Read the model definition and answer for the solid it produces. Units are mm, in the model's axes. Coordinates: 2 decimals unless noted, no trailing zeros. Write each loop counter-clockwise with the first axis right and the second up, starting at its lowest first coordinate (ties: lowest second). Pieces come first, ordered by that corner, then holes. Notation, with made-up numbers: (45.5, 1.5) -> (93.5, 1.5) arc R35 ccw to (93.5, 38.5) -> close; hole circle Ø8 at (17, 55.5). An arc over 180 degrees is marked (long way). Write item = value, one per line. Start each with the question number.
1) For a pull along Y with two mould halves and no side action, classify faces 1 (the face through (9, 0, 3.175)), 2 (the face through (13.45, 0.24, 1.61)), 3 (the face through (26.034, 0.092, 1.565)) as released by +Y, released by -Y, zero draft, split by the parting line, or undercut.
2) Section D-D (y = -2.25) is taken. Determine the outline of the cut face in (x, z) (3 decimals).
3) Section A-A (z = 2.6) is taken. Determine the outline of the cut face in (x, y).
4) Flat-ended cylindrical pins translate along their axes: pin 1 Ø1.4 at (x, y) = (18.796, 0) entering from +Z; pin 2 Ø3 at (x, y) = (19, 0.5) entering from -Z; pin 3 Ø1.5 at (x, z) = (7.5, 2.5) entering from +Y. Find the tip coordinate at first contact, or state that the pin passes through.
5) Find the intervals of material crossed by line 1 along Y through (x, z) = (12.7, 1); line 2 along X through (y, z) = (-1, 2.6); line 3 along Y through (x, z) = (-2, 1.05), in increasing order. Write a range as from..to.
6) Section C-C (x = 12.5) is taken. Determine the outline of the cut face in (y, z) (3 decimals), plus the area to 3 significant figures.
7) Section B-B (y = 0) is taken. Determine the outline of the cut face in (x, z) (3 decimals), plus the area to 3 significant figures.
Autodesk Inventor part; units mm, degrees
ref_plane "YZ Plane" through (0, 0, 0) normal (1, 0, 0) x (0, 1, 0)
ref_plane "XZ Plane" through (0, 0, 0) normal (0, 1, 0) x (-1, 0, 0)
ref_plane "XY Plane" through (0, 0, 0) normal (0, 0, 1) x (1, 0, 0)
sketch "Sketch1" plane through (0, 0, 0) normal (0, 0, 1) x (1, 0, 0)
  circle A0 centre (0, 0) radius 6.9469
  circle A1 centre (21.844, 0) radius 4.191
  line L0 (0, 6.9469) -> (21.844, 4.191)
  line L1 (0, -6.9469) -> (21.844, -4.191)
  dimension "d0" = 13.8938
  dimension "d1" = 8.382
  dimension "d2" = 21.844
extrude "Extrusion1" add sketch "Sketch1" along normal blind 3.175 contours L0 A0 L1 | L0 A1 L1 A0 | A1
sketch "Sketch2" plane through (0, 0, 3.175) normal (0, 0, 1) x (1, 0, 0)
  circle A0 centre (0, 0) radius 2.54
  circle A1 centre (12.7, 0) radius 0.7874
  circle A2 centre (15.748, 0) radius 0.7874
  circle A3 centre (18.796, 0) radius 0.7874
  circle A4 centre (21.844, 0) radius 0.7874
  dimension "d5" = 5.08
  dimension "d6" = 1.5748
  dimension "d7" = 1.5748
  dimension "d8" = 1.5748
  dimension "d9" = 1.5748
  dimension "d10" = 12.7
  dimension "d11" = 15.748
  dimension "d12" = 18.796
  dimension "d13" = 21.844
extrude "Extrusion2" cut sketch "Sketch2" against normal blind 3.175
properties part number "Servo horn"
Answer key:
q1.face_1 = zero draft
q1.face_2 = undercut
q1.face_3 = split by the parting line
q2.outline = (-6.572, 0) -> (-1.179, 0) -> (-1.179, 3.175) -> (-6.572, 3.175) -> close; (1.179, 0) -> (25.38, 0) -> (25.38, 3.175) -> (1.179, 3.175) -> close
q3.outline = (0, -6.95) -> (21.84, -4.19) arc R4.19 ccw to (21.84, 4.19) -> (0, 6.95) arc R6.95 ccw to start; hole circle Ø5.08 at (0, 0); hole circle Ø1.57 at (12.7, 0); hole circle Ø1.57 at (15.75, 0); hole circle Ø1.57 at (18.8, 0); hole circle Ø1.57 at (21.84, 0)
q4.pin_1 = through
q4.pin_2 = 0
q4.pin_3 = 6.1
q5.line_1 = -5.34..-0.79, 0.79..5.34
q5.line_2 = -6.87..-2.33, 2.33..25.91
q5.line_3 = -6.65..-1.57, 1.57..6.65
q6.outline = (-5.37, 0) -> (-0.762, 0) -> (-0.762, 3.175) -> (-5.37, 3.175) -> close; (0.762, 0) -> (5.37, 0) -> (5.37, 3.175) -> (0.762, 3.175) -> close
q6.area = 29.3 mm^2
q7.outline = (-6.947, 0) -> (-2.54, 0) -> (-2.54, 3.175) -> (-6.947, 3.175) -> close; (2.54, 0) -> (11.913, 0) -> (11.913, 3.175) -> (2.54, 3.175) -> close; (13.487, 0) -> (14.961, 0) -> (14.961, 3.175) -> (13.487, 3.175) -> close; (16.535, 0) -> (18.009, 0) -> (18.009, 3.175) -> (16.535, 3.175) -> close; (19.583, 0) -> (21.057, 0) -> (21.057, 3.175) -> (19.583, 3.175) -> close; (22.631, 0) -> (26.035, 0) -> (26.035, 3.175) -> (22.631, 3.175) -> close
q7.area = 68.6 mm^2
